Verification items for the finished model (mm, model axes). Round coordinates to 2 decimals unless told otherwise and drop trailing zeros. Order: outer loops, then holes, each group sorted by start corner. A loop starts at its lowest first (then second) coordinate and runs counter-clockwise, first axis right, second up. Notation, with made-up numbers: (67.5, 63.25) -> (110.5, 63.25) arc R10 ccw to (110.5, 67.25) -> close; hole circle Ø3 at (-28, 30.25). An arc over 180 degrees is marked (long way). Return JSON: item names as keys, results as strings. Group by question number.
1) Section check A-A on x = -133.35. Enter the section's corners in (y, z) (3 decimals).
2) Section check B-B on x = -10.5. Enter the section's corners in (y, z).
3) Depth check by flat-ended pin: pin 1 (1 mm diameter, centred on x = 10.5, z = 5, fed in from +Y). Enter the tip coordinate at first touch or a pass-through.
4) Scan lines: L1, parallel to Y at x = -164, z = 11.25; L2, parallel to Y at x = 45.5, z = 11.5. Record each from-to range of solid material in increasing order.
```python
from build123d import *

# Parameters (mm, degrees)
SKETCH1_W           = 381
SKETCH1_H           = 25.4
BOSS_EXTRUDE1_DEPTH = 12.7
CUT_EXTRUDE1_REACH  = 194.605
SKETCH2_R           = 4.445
LPATTERN1_COUNT     = 37
LPATTERN1_PITCH     = 10.16


with BuildPart() as part:
    # Sketch1 → Boss-Extrude1 (new body)
    with BuildSketch(Plane.XY):
        with Locations((0, 12.7)):
            Rectangle(SKETCH1_W, SKETCH1_H)
    extrude(amount=BOSS_EXTRUDE1_DEPTH)

    # Sketch2 → Cut-Extrude1 (cut, up to next)
    with BuildSketch(Plane.XY.offset(12.7), mode=Mode.PRIVATE) as cut_extrude1_sk1:
        with Locations((-184.15, 25.4)):
            Circle(SKETCH2_R)
    cut_extrude1_tool1 = extrude(cut_extrude1_sk1.sketch, amount=-CUT_EXTRUDE1_REACH, mode=Mode.PRIVATE) & part.part
    cut_extrude1 = cut_extrude1_tool1.solids().sort_by_distance((-184.15, 25.4, 12.7))[0]
    add(cut_extrude1, mode=Mode.SUBTRACT)

    # LPattern1: Cut-Extrude1 ×37
    with Locations(*[(i * LPATTERN1_PITCH, 0, 0) for i in range(1, LPATTERN1_COUNT)]):
        add(cut_extrude1, mode=Mode.SUBTRACT)


solid = part.part
```
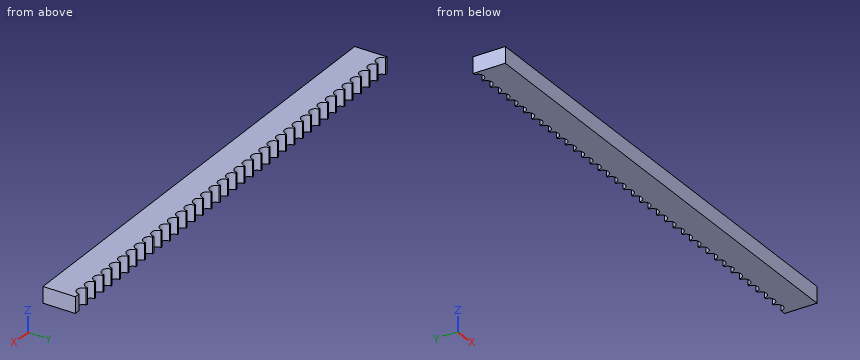
Check result:
{
 "1": {"outline": "(0, 0) -> (20.955, 0) -> (20.955, 12.7) -> (0, 12.7) -> close"},
 "2": {"outline": "(0, 0) -> (21.05, 0) -> (21.05, 12.7) -> (0, 12.7) -> close"},
 "3": {"pin 1": "y = 21.49"},
 "4": {"L1": "0 to 20.96", "L2": "0 to 23.52"}
}
